Source: CAD feature listing. Evaluate the final solid. Frame: model axes, mm. A direction names the side the tool comes from. Round coordinates to 2 decimals unless told otherwise and drop trailing zeros. Loops run counter-clockwise (first coordinate to the right, second up) from the corner with the lowest first, then second, coordinate; pieces in that order, holes last. Notation, with made-up numbers: (75, 82.5) - (122, 82.5) arc R14 cw to (122, 92.5) - close; hole circle Ø11 at (22.5, -10). An arc over 180 degrees is marked (long way). Use CSV: the item, a comma, the result in double quotes. Start each with the question number.
from build123d import *

# Parameters (mm, degrees)
SKETCH1_W                      = 89.225
SKETCH1_H                      = 307.5
SKETCH1_W_2                    = 69.225
SKETCH1_H_2                    = 42
SKETCH1_H_3                    = 20
SKETCH1_H_4                    = 51
SKETCH1_H_5                    = 14.3
SKETCH1_H_6                    = 25
BOSS_EXTRUDE1_DEPTH            = 2
SKETCH20_W                     = 22
SKETCH20_H                     = 1
BOSS_EXTRUDE7_DEPTH            = 2
SKETCH21_W                     = 22
SKETCH21_H                     = 2
BOSS_EXTRUDE8_DEPTH            = 12
FILLET7_R                      = 2
FILLET8_R                      = 1
M2_5_CLEARANCE_HOLE3_D         = 2.9
SKETCH28_W                     = 12
SKETCH28_H                     = 1
BOSS_EXTRUDE11_DEPTH           = 2
SKETCH29_W                     = 12
SKETCH29_H                     = 2
BOSS_EXTRUDE12_DEPTH           = 12
FILLET11_R                     = 2
FILLET12_R                     = 1
M2_5_START                     = -286.2
M2_5_CLEARANCE_HOLE5_OUTLINE_R = 1.45
M2_5_CLEARANCE_HOLE5_DEPTH     = 80
M2_5_CLEARANCE_HOLE6_D         = 2.9
M2_CLEARANCE_HOLE1_D           = 2.4


# Read off the part's stored shape, not the designer's step: M2.5 Clearance Hole5
with BuildPart() as part:
    # Sketch1 → Boss-Extrude1 (new body)
    with BuildSketch(Plane(origin=(0, 0, 0), x_dir=(1, 0, 0), z_dir=(0, 1, 0))):
        with Locations((44.6125, 153.75)):
            Rectangle(SKETCH1_W, SKETCH1_H)
        with Locations((44.6125, 246.2)):
            Rectangle(SKETCH1_W_2, SKETCH1_H_2, mode=Mode.SUBTRACT)
        Polygon((10, 10), (79.225, 10), (79.225, 21.8), (56.6125, 21.8), (32.6125, 21.8), (10, 21.8), align=None, mode=Mode.SUBTRACT)
        Polygon((10, 27.8), (79.225, 27.8), (79.225, 39.6), (56.6125, 39.6), (32.6125, 39.6), (10, 39.6), align=None, mode=Mode.SUBTRACT)
        Polygon((10, 45.6), (79.225, 45.6), (79.225, 57.4), (56.6125, 57.4), (32.6125, 57.4), (10, 57.4), align=None, mode=Mode.SUBTRACT)
        Polygon((10, 63.4), (79.225, 63.4), (79.225, 75.2), (56.6125, 75.2), (32.6125, 75.2), (10, 75.2), align=None, mode=Mode.SUBTRACT)
        with Locations((44.6125, 91.2)):
            Rectangle(SKETCH1_W_2, SKETCH1_H_3, mode=Mode.SUBTRACT)
        with Locations((44.6125, 142.7)):
            Rectangle(SKETCH1_W_2, SKETCH1_H_4, mode=Mode.SUBTRACT)
        with Locations((44.6125, 290.35)):
            Rectangle(SKETCH1_W_2, SKETCH1_H_5, mode=Mode.SUBTRACT)
        with Locations((44.6125, 196.7)):
            Rectangle(SKETCH1_W_2, SKETCH1_H_6, mode=Mode.SUBTRACT)
    extrude(amount=BOSS_EXTRUDE1_DEPTH)

    # Sketch20 → Boss-Extrude7 (add)
    with BuildSketch(Plane(origin=(0, 0, 0), x_dir=(1, 0, 0), z_dir=(0, 1, 0))):
        with Locations((33.7, 184.7)):
            Rectangle(SKETCH20_W, SKETCH20_H)
    extrude(amount=BOSS_EXTRUDE7_DEPTH)

    # Sketch21 → Boss-Extrude8 (add)
    with BuildSketch(Plane(origin=(0, 0, 0), x_dir=(1, 0, 0), z_dir=(0, 1, 0))):
        with Locations((33.7, 186.2)):
            Rectangle(SKETCH21_W, SKETCH21_H)
    extrude(amount=BOSS_EXTRUDE8_DEPTH)

    # Fillet7
    fillet7_edges = [part.edges().sort_by_distance(p)[0] for p in [
        (33.7, 0, -187.2),
    ]]
    fillet(fillet7_edges, radius=FILLET7_R)

    # Fillet8
    fillet8_edges = [part.edges().sort_by_distance(p)[0] for p in [
        (33.7, 2, -185.2),
    ]]
    fillet(fillet8_edges, radius=FILLET8_R)

    # M2.5 Clearance Hole3 (through all)
    with Locations(Plane.XY.offset(-185.2)):
        with Locations((33.7, 7.4125)):
            Hole(M2_5_CLEARANCE_HOLE3_D / 2)

    # Sketch28 → Boss-Extrude11 (add)
    with BuildSketch(Plane(origin=(0, 0, 0), x_dir=(1, 0, 0), z_dir=(0, 1, 0))):
        with Locations((66.6125, 208.7)):
            Rectangle(SKETCH28_W, SKETCH28_H)
        with Locations((44.6125, 208.7)):
            Rectangle(SKETCH28_W, SKETCH28_H)
        with Locations((22.6125, 208.7)):
            Rectangle(SKETCH28_W, SKETCH28_H)
        with Locations((66.6125, 283.7)):
            Rectangle(SKETCH28_W, SKETCH28_H)
        with Locations((44.6125, 283.7)):
            Rectangle(SKETCH28_W, SKETCH28_H)
        with Locations((22.6125, 283.7)):
            Rectangle(SKETCH28_W, SKETCH28_H)
    extrude(amount=BOSS_EXTRUDE11_DEPTH)

    # Sketch29 → Boss-Extrude12 (add)
    with BuildSketch(Plane(origin=(0, 0, 0), x_dir=(1, 0, 0), z_dir=(0, 1, 0))):
        with Locations((66.6125, 207.2)):
            Rectangle(SKETCH29_W, SKETCH29_H)
        with Locations((44.6125, 207.2)):
            Rectangle(SKETCH29_W, SKETCH29_H)
        with Locations((22.6125, 207.2)):
            Rectangle(SKETCH29_W, SKETCH29_H)
        with Locations((66.6125, 285.2)):
            Rectangle(SKETCH29_W, SKETCH29_H)
        with Locations((44.6125, 285.2)):
            Rectangle(SKETCH29_W, SKETCH29_H)
        with Locations((22.6125, 285.2)):
            Rectangle(SKETCH29_W, SKETCH29_H)
    extrude(amount=BOSS_EXTRUDE12_DEPTH)

    # Fillet11
    fillet11_edges = [part.edges().sort_by_distance(p)[0] for p in [
        (66.6125, 0, -206.2),
        (44.6125, 0, -206.2),
        (22.6125, 0, -206.2),
        (66.6125, 0, -286.2),
        (44.6125, 0, -286.2),
        (22.6125, 0, -286.2),
    ]]
    fillet(fillet11_edges, radius=FILLET11_R)

    # Fillet12
    fillet12_edges = [part.edges().sort_by_distance(p)[0] for p in [
        (22.6125, 2, -284.2),
        (44.6125, 2, -284.2),
        (66.6125, 2, -284.2),
        (66.6125, 2, -208.2),
        (44.6125, 2, -208.2),
        (22.6125, 2, -208.2),
    ]]
    fillet(fillet12_edges, radius=FILLET12_R)

    # M2.5 Clearance Hole5 outline → M2.5 Clearance Hole5 (cut)
    with BuildSketch(Plane.XY.offset(M2_5_START)):
        with Locations((22.6125, 9.5)):
            Circle(M2_5_CLEARANCE_HOLE5_OUTLINE_R)
        with Locations((44.6125, 9.5)):
            Circle(M2_5_CLEARANCE_HOLE5_OUTLINE_R)
        with Locations((66.6125, 9.5)):
            Circle(M2_5_CLEARANCE_HOLE5_OUTLINE_R)
    extrude(amount=M2_5_CLEARANCE_HOLE5_DEPTH, mode=Mode.SUBTRACT)

    # M2.5 Clearance Hole6 (through all)
    with Locations(Plane(origin=(0, 2, 0), x_dir=(1, 0, 0), z_dir=(0, 1, 0))):
        with Locations((85.025, 4), (4.2, 4), (4.2, 109.2), (4.2, 176.2), (4.2, 303.5), (85.025, 303.5), (85.025, 176.2), (85.025, 109.2)):
            Hole(M2_5_CLEARANCE_HOLE6_D / 2)

    # M2 Clearance Hole1 (through all)
    with Locations(Plane(origin=(0, 0, 0), x_dir=(-1, 0, 0), z_dir=(0, -1, 0))):
        with Locations((-44.6125, 24.8), (-44.6125, 42.9), (-44.6125, 60.4), (-44.6125, 78.2)):
            Hole(M2_CLEARANCE_HOLE1_D / 2)


solid = part.part
1. Section query A-A on z = -124.5. Return the cut outline in (x, y) (3 decimals).
2. Contact query for flat-ended pins moving along their axis: P1, Ø7, axis at x = 30.5, y = 7, coming from the +Z side; P2, Ø0.9, axis at y = 6.5, z = -207, coming from the +X side; P3, Ø2.5, axis at x = 65.5, y = 6.5, coming from the +Z side. Output: stop coordinate, or through.
3. Mould query, pull axis Z, two halves, no side actions, for faces 1 (the flat face through (41, 0, -177)), 2 (the flat face through (23, 7, -286.2)), 3 (the flat face through (45, 7, -284.2)). Classes: +Z half, -Z half, draft (parallel to the pull), parting line (faces both ways), or undercut.
4. Line query: line 1 along X through (y, z) = (1.5, -78.5) (3 decimals); line 2 along X through (y, z) = (9.5, -207.8); line 3 along Z through (x, y) = (25, 6.5). Output: solid intervals per line, ascending.
5. Reachability of faces 4 (the flat face through (34, 9, -185.2)), 5 (the flat face through (67, 7, -206.2)), 6 (the flat face through (45, 7, -206.2)), 7 (the flat face through (23, 7, -284.2)), 8 (the flat face through (67, 7, -286.2)) from +Z, -Z, +X, -X, +Y, -Y: full face, straight path, thin tool, end or side. Return the list, or none.
6. Section query B-B on z = -275.5. Return the cut outline in (x, y) (3 decimals), and give its area (3 significant figures).
Values:
1,outline,"(0, 0) - (10, 0) - (10, 2) - (0, 2) - close; (79.225, 0) - (89.225, 0) - (89.225, 2) - (79.225, 2) - close"
2,P1,"stops at z = -185.2"
2,P2,"stops at x = 72.61"
2,P3,"stops at z = -206.2"
3,face 1,"draft"
3,face 2,"-Z half"
3,face 3,"undercut"
4,line 1,"x = 0 to 43.451, 45.774 to 89.225"
4,line 2,"x = 16.61 to 21.16, 24.06 to 28.61, 38.61 to 43.16, 46.06 to 50.61, 60.61 to 65.16, 68.06 to 72.61"
4,line 3,"z = -286.2 to -284.2, -208.2 to -206.2, -187.2 to -185.2"
5,face 4,"+Z, +X, -X, +Y"
5,face 5,"+Z, +X, -X, +Y, -Y"
5,face 6,"+X, -X, +Y, -Y"
5,face 7,"+X, -X, +Y"
5,face 8,"-Z, +X, -X, +Y, -Y"
6,outline,"(0, 0) - (89.225, 0) - (89.225, 2) - (0, 2) - close"
6,area,"178 mm^2"
